from build123d import *

# Parameters (mm, degrees)
F0_R     = 30.5
F0_R_2   = 15.25
F1_DEPTH = 4
F2_R     = 25.75
F2_R_2   = 15.25
F3_DEPTH = 6
F4_SIZE  = 1
F5_SIZE  = 1


with BuildPart() as f1:
    # F0 (on Top) → F1 (new body)
    with BuildSketch(Plane.XY):
        Circle(F0_R)
        Circle(F0_R_2, mode=Mode.SUBTRACT)
    extrude(amount=F1_DEPTH)

    # F2 (on face) → F3 (join)
    with BuildSketch(Plane.XY.offset(4)):
        Circle(F2_R)
        Circle(F2_R_2, mode=Mode.SUBTRACT)
    extrude(amount=F3_DEPTH)

    # F4
    f4_edges = [f1.edges().sort_by_distance(p)[0] for p in [
        (-25.75, 0, 10),
        (-30.5, 0, 4),
    ]]
    chamfer(f4_edges, length=F4_SIZE)

    # F5
    f5_edges = [f1.edges().sort_by_distance(p)[0] for p in [
        (-15.25, 0, 0),
    ]]
    chamfer(f5_edges, length=F5_SIZE)


solid = f1.part
Check sheet for the modelled part. Datum: model origin and axes. Units: mm. A direction names the side the tool comes from. Coordinates: 2 decimals unless noted, no trailing zeros. Write each loop counter-clockwise with the first axis right and the second up, starting at its lowest first coordinate (ties: lowest second). Pieces come first, ordered by that corner, then holes. Notation, with made-up numbers: M 53,32.5 L 91,32.5 A13 cw 91,40.5 Z; hole C 33,-5.75 d9. An arc over 180 degrees is marked long. Answer as CSV lines item,"result".
Q1. Cross-section at A-A (y = 0). Record the boundary of the cut face in (x, z).
Check result:
outline,"M -30.5,0 L -16.25,0 L -15.25,1 L -15.25,10 L -24.75,10 L -25.75,9 L -25.75,4 L -29.5,4 L -30.5,3 Z; M 15.25,1 L 16.25,0 L 30.5,0 L 30.5,3 L 29.5,4 L 25.75,4 L 25.75,9 L 24.75,10 L 15.25,10 Z"
Q2. Mould release check, pull along Y, two halves, no side actions. Record for faces 1 (the face through (-5.58, -25.14, 6.46)), 2 (the face through (13, -13, 0)), 3 (the face through (-12.1, -9.28, 5.44)): released by +Y, released by -Y, zero draft, split by the parting line, or undercut.
Check result:
face 1,"split by the parting line"
face 2,"zero draft"
face 3,"undercut"
Q3. Go/stop test with flat-tipped pins: pin 1 (1 mm diameter, centred on y = 18.5, z = 8.5, fed in from +X); pin 2 (4 mm diameter, centred on y = 10.5, z = 5.5, fed in from +X); pin 3 (1.5 mm diameter, centred on y = 17.5, z = 8.5, fed in from +X); pin 4 (6 mm diameter, centred on x = -20.5, y = -15.5, fed in from +Z). Record where each tip stops, or that it passes through.
Check result:
pin 1,"x = 18.41"
pin 2,"x = 28.22"
pin 3,"x = 19.56"
pin 4,"z = 10"
Q4. Material ranges on probe 1 along Y at (x, z) = (0, 5); probe 2 along X at (y, z) = (-0.5, 2.25); probe 3 along X at (y, z) = (10.5, 6), recorded low to high. Write a range as from..to.
Check result:
probe 1,"-25.75..-15.25, 15.25..25.75"
probe 2,"-30.5..-15.24, 15.24..30.5"
probe 3,"-23.51..-11.06, 11.06..23.51"
Q5. Cross-section at C-C (z = 6). Record the boundary of the cut face in (x, y).
Check result:
outline,"C 0,0 d51.5; hole C 0,0 d30.5"
Q6. Set-up check for faces 4 (the face through (2, 26, 4)), 5 (the face through (-24.204, -18.559, 1.479)): record each of +Z, -Z, +X, -X, +Y, -Y from which the full face is reachable in a straight line by a thin tool's end or side.
Check result:
face 4,"+Z"
face 5,"+Z, -Z"
